The listing builds one solid part. Answer for the finished solid, in the listing's coordinates (mm). Face numbers are marked on the shaded views. A direction names the side the tool comes from. Coordinates: 2 decimals unless noted, no trailing zeros. Order: outer loops, then holes, each group sorted by start corner. A loop starts at its lowest first (then second) coordinate and runs counter-clockwise, first axis right, second up. Notation, with made-up numbers: (-11.5, 89.25) -> (12.5, 89.25) arc R25 ccw to (12.5, 126.25) -> close; hole circle Ø2 at (56, 57). An arc over 180 degrees is marked (long way). Return JSON: item names as keys, results as strings.
```python
from build123d import *

# Parameters (mm, degrees)
CORTE_EXTRUS_O1_DEPTH = 1.5


with BuildPart() as part:
    # Esboço1 → Revolução1 (revolve)
    with BuildSketch(Plane(origin=(0, 0, 0), x_dir=(1, 0, 0), z_dir=(0, 1, 0))):
        Polygon((0, 0), (2.75, 0), (2.75, -3), (1.5, -3), (1.5, -13), (0, -13), (0, -3), align=None)
    revolve(axis=Axis((0, 0, 3), (0, 0, -1)))

    # Esboço2 → Corte-extrusão1 (cut)
    with BuildSketch(Plane(origin=(0, 0, 0), x_dir=(-1, 0, 0), z_dir=(0, 0, -1))):
        Polygon((1.732050808, 0), (0.866025404, 1.5), (-0.866025404, 1.5), (-1.732050808, 0), (-0.866025404, -1.5), (0.866025404, -1.5), align=None)
    extrude(amount=-CORTE_EXTRUS_O1_DEPTH, mode=Mode.SUBTRACT)


solid = part.part
```
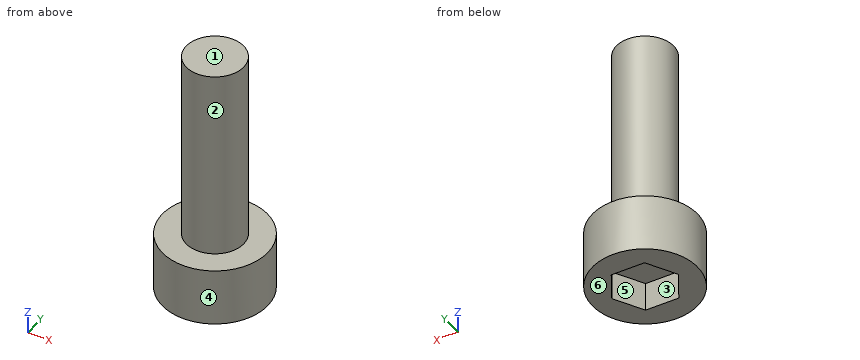
Item 1: The part is cut by section B-B on y = 1.25. Determine the outline of the cut face in (x, z).
Answer list:
{"outline": "(-2.45, 0) -> (-1.01, 0) -> (-1.01, 1.5) -> (1.01, 1.5) -> (1.01, 0) -> (2.45, 0) -> (2.45, 3) -> (0.83, 3) -> (0.83, 13) -> (-0.83, 13) -> (-0.83, 3) -> (-2.45, 3) -> close"}
Item 2: The part is cut by section D-D on z = 6.75. Determine the outline of the cut face in (x, y).
Answer list:
{"outline": "circle Ø3 at (0, 0)"}
Item 3: Find the intervals of material crossed by probe 1 along Z at (x, y) = (-0.5, -1.7); probe 2 along Z at (x, y) = (1.35, 0.3); probe 3 along Y at (x, z) = (1.3, 1.25), in increasing order.
Answer list:
{"probe 1": "0 to 3", "probe 2": "1.5 to 13", "probe 3": "-2.42 to -0.75, 0.75 to 2.42"}
Item 4: Flat-ended cylindrical pins translate along their axes: pin 1 (0.9 mm diameter, centred on x = 0, y = 0.5, fed in from -Z); pin 2 (1.6 mm diameter, centred on x = -1.5, y = 0.5, fed in from +Z); pin 3 (1 mm diameter, centred on x = -0.5, z = 8, fed in from -Y). Find the tip coordinate at first contact, or state that the pin passes through.
Answer list:
{"pin 1": "z = 1.5", "pin 2": "z = 13", "pin 3": "y = -1.5"}
Item 5: Determine the mould class of the marked faces 4, 5 and 6 for opening direction X: pulls with the +X half, pulls with the -X half, needs draft (parallel to the pull), parting line crosses it, or undercut.
Answer list:
{"face 4": "parting line crosses it", "face 5": "undercut", "face 6": "needs draft"}
Item 6: Which of the six approach directions +Z, -Z, +X, -X, +Y, -Y give full straight-line access (tool end or side, diameter ignored) to the marked faces 1, 2 and 3?
Answer list:
{"face 1": "+Z, +X, -X, +Y, -Y", "face 2": "+Z", "face 3": "-Z"}
Item 7: The part is cut by section C-C on z = 2. Determine the outline of the cut face in (x, y).
Answer list:
{"outline": "circle Ø5.5 at (0, 0)"}
Item 8: The part is cut by section A-A on x = 0. Determine the outline of the cut face in (y, z).
Answer list:
{"outline": "(-2.75, 0) -> (-1.5, 0) -> (-1.5, 1.5) -> (1.5, 1.5) -> (1.5, 0) -> (2.75, 0) -> (2.75, 3) -> (1.5, 3) -> (1.5, 13) -> (-1.5, 13) -> (-1.5, 3) -> (-2.75, 3) -> close"}
